Check sheet for the modelled part. Datum: model origin and axes. Units: mm. A direction names the side the tool comes from. Round coordinates to 2 decimals unless told otherwise and drop trailing zeros. Order: outer loops, then holes, each group sorted by start corner. A loop starts at its lowest first (then second) coordinate and runs counter-clockwise, first axis right, second up. Notation, with made-up numbers: (76.5, 6.5) -> (114.5, 6.5) arc R21 cw to (114.5, 14.5) -> close; hole circle Ø4 at (56.25, -19). An arc over 180 degrees is marked (long way). Answer in a Markdown table with one row per item.
```python
from build123d import *

# Parameters (mm, degrees)
F0_W         = 31
F0_H         = 21
F1_DEPTH     = 28
F2_W         = 21
F2_H         = 42
F3_DEPTH     = 50.8
F4_DEPTH     = 25.4
F6_DEPTH     = 25.4
F7_DEPTH     = 25.4
F8_DEPTH     = 2
F9_W         = 10.5
F9_H         = 2
F10_DEPTH    = 10.5
F11_DEPTH    = 10.5
F12_W        = 18.7637824565
F12_H        = 49.8975180089
F13_DEPTH    = 25.4
F14_DEPTH    = 25.4
F15_DEPTH    = 0.25
F16_DEPTH    = 0.25
F17_DEPTH    = 1
F18_T1_DEPTH = 46.4


# Not quite as in the source:
# - a fillet or chamfer that OpenCascade refuses, or shapes differently, is made with other operations: its cross-section is extruded or revolved along the edge and cut away or added


with BuildPart() as f1:
    # F0 (on Top) → F1 (new body)
    with BuildSketch(Plane.XY):
        Rectangle(F0_W, F0_H)
    extrude(amount=F1_DEPTH)

    # F2 (on Front) → F3 (cut)
    with BuildSketch(Plane.XZ):
        Rectangle(F2_W, F2_H)
    extrude(amount=-F3_DEPTH, mode=Mode.SUBTRACT)

    # F2 (on Front) → F4 (cut)
    with BuildSketch(Plane.XZ):
        Rectangle(F2_W, F2_H)
    extrude(amount=F4_DEPTH, mode=Mode.SUBTRACT)

    # F5 (on Right) → F6 (cut)
    with BuildSketch(Plane.YZ):
        with BuildLine():
            Line((0, 24.5501343161), (2.5, 24.5501343161))
            ThreePointArc((2.5, 24.5501343161), (0, 27.0501343161), (-2.5, 24.5501343161))
            Line((-2.5, 24.5501343161), (0, 24.5501343161))
        make_face()
        with BuildLine():
            Line((2.5, -28.5555105656), (2.5, 24.5501343161))
            ThreePointArc((2.5, 24.5501343161), (1.767766953, 22.7823673631), (0, 22.0501343161))
            Line((0, 22.0501343161), (0, -28.5555105656))
            Line((0, -28.5555105656), (2.5, -28.5555105656))
        make_face()
        with BuildLine():
            ThreePointArc((0, 22.0501343161), (1.767766953, 22.7823673631), (2.5, 24.5501343161))
            Line((2.5, 24.5501343161), (0, 24.5501343161))
            Line((0, 24.5501343161), (0, 22.0501343161))
        make_face()
        with BuildLine():
            Line((0, 24.5501343161), (-2.5, 24.5501343161))
            ThreePointArc((-2.5, 24.5501343161), (-1.767766953, 22.7823673631), (0, 22.0501343161))
            Line((0, 22.0501343161), (0, 24.5501343161))
        make_face()
        with BuildLine():
            ThreePointArc((0, 22.0501343161), (-1.767766953, 22.7823673631), (-2.5, 24.5501343161))
            Line((-2.5, 24.5501343161), (-2.5, -33.7370373309))
            Line((-2.5, -33.7370373309), (0, -33.7370373309))
            Line((0, -33.7370373309), (0, -28.5555105656))
            Line((0, -28.5555105656), (0, 22.0501343161))
        make_face()
    extrude(amount=-F6_DEPTH, mode=Mode.SUBTRACT)

    # F5 (on Right) → F7 (cut)
    with BuildSketch(Plane.YZ):
        with BuildLine():
            Line((0, 24.5501343161), (2.5, 24.5501343161))
            ThreePointArc((2.5, 24.5501343161), (0, 27.0501343161), (-2.5, 24.5501343161))
            Line((-2.5, 24.5501343161), (0, 24.5501343161))
        make_face()
        with BuildLine():
            Line((2.5, -28.5555105656), (2.5, 24.5501343161))
            ThreePointArc((2.5, 24.5501343161), (1.767766953, 22.7823673631), (0, 22.0501343161))
            Line((0, 22.0501343161), (0, -28.5555105656))
            Line((0, -28.5555105656), (2.5, -28.5555105656))
        make_face()
        with BuildLine():
            ThreePointArc((0, 22.0501343161), (1.767766953, 22.7823673631), (2.5, 24.5501343161))
            Line((2.5, 24.5501343161), (0, 24.5501343161))
            Line((0, 24.5501343161), (0, 22.0501343161))
        make_face()
        with BuildLine():
            Line((0, 24.5501343161), (-2.5, 24.5501343161))
            ThreePointArc((-2.5, 24.5501343161), (-1.767766953, 22.7823673631), (0, 22.0501343161))
            Line((0, 22.0501343161), (0, 24.5501343161))
        make_face()
        with BuildLine():
            ThreePointArc((0, 22.0501343161), (-1.767766953, 22.7823673631), (-2.5, 24.5501343161))
            Line((-2.5, 24.5501343161), (-2.5, -33.7370373309))
            Line((-2.5, -33.7370373309), (0, -33.7370373309))
            Line((0, -33.7370373309), (0, -28.5555105656))
            Line((0, -28.5555105656), (0, 22.0501343161))
        make_face()
    extrude(amount=F7_DEPTH, mode=Mode.SUBTRACT)

    # F8 (add): faces of the model
    f8_faces = [f1.faces().sort_by_distance(p)[0] for p in [
        (13, 6.5, 0),
        (13, -6.5, 0),
        (-13, -6.5, 0),
        (-13, 6.5, 0),
    ]]
    extrude(f8_faces, amount=F8_DEPTH)

    # F9 (on Right) → F10 (join)
    with BuildSketch(Plane.YZ):
        with Locations((-5.25, -1)):
            Rectangle(F9_W, F9_H)
        with Locations((5.25, -1)):
            Rectangle(F9_W, F9_H)
    extrude(amount=F10_DEPTH)

    # F11 (add): a face of the model
    f11_faces = [f1.faces().sort_by_distance(p)[0] for p in [
        (0, 0, -1),
    ]]
    extrude(f11_faces, amount=F11_DEPTH)

    # F12 (on Top) → F13 (cut)
    with BuildSketch(Plane.XY):
        Rectangle(F12_W, F12_H)
    extrude(amount=-F13_DEPTH, mode=Mode.SUBTRACT)

    # F14 (cut): a face of the model
    f14_faces = [f1.faces().sort_by_distance(p)[0] for p in [
        (10.5, 0, -1),
    ]]
    extrude(f14_faces, amount=-F14_DEPTH, mode=Mode.SUBTRACT)

    # F15 (add): faces of the model
    f15_faces = [f1.faces().sort_by_distance(p)[0] for p in [
        (9.3818912283, 6.5, -1),
        (9.3818912283, -6.5, -1),
    ]]
    extrude(f15_faces, amount=F15_DEPTH)

    # F16 (add): faces of the model
    f16_faces = [f1.faces().sort_by_distance(p)[0] for p in [
        (-9.3818912283, 6.5, -1),
        (-9.3818912283, -6.5, -1),
    ]]
    extrude(f16_faces, amount=F16_DEPTH)

    # F17 (add): a face of the model
    f17_faces = [f1.faces().sort_by_distance(p)[0] for p in [
        (0, 0, 28),
    ]]
    extrude(f17_faces, amount=F17_DEPTH)

    # F18: fillet of radius 5.08 on 2 edges, made by hand

    # F18_s2 → F18_t1 (cut)
    with BuildSketch(Plane.XZ.offset(-23.2)):
        with BuildLine():
            ThreePointArc((-15.5, 23.92), (-14.0121024484, 27.5121024484), (-10.42, 29))
            Line((-10.42, 29), (-15.5, 29))
            Line((-15.5, 29), (-15.5, 23.92))
        make_face()
        with BuildLine():
            ThreePointArc((15.5, 23.92), (14.0121024484, 27.5121024484), (10.42, 29))
            Line((10.42, 29), (15.5, 29))
            Line((15.5, 29), (15.5, 23.92))
        make_face()
    extrude(amount=F18_T1_DEPTH, mode=Mode.SUBTRACT)


solid = f1.part
```
(1) Section check D-D on x = -2. Record the boundary of the cut face in (y, z), plus the area to 3 significant figures.
Solutions:
| item | result |
|---|---|
| outline | (-10.5, 21) -> (-2.5, 21) -> (-2.5, 24.55) arc R2.5 cw to (2.5, 24.55) -> (2.5, 21) -> (10.5, 21) -> (10.5, 29) -> (-10.5, 29) -> close |
| area | 140 mm^2 |
(2) Tool access check on faces 5 (the flat face through (10, 6, 0)), 6 (the flat face through (0, 0, 29)), 7 (the flat face through (9.132, -7, -1)). Record the directions out of +Z, -Z, +X, -X, +Y, -Y that give a thin tool (end or side, any length) a straight path to the whole face; none if there is none.
Solutions:
| item | result |
|---|---|
| face 5 | +Y, -Y |
| face 6 | +Z, +X, -X, +Y, -Y |
| face 7 | -Z, +Y, -Y |
(3) Scan lines: probe 1 along Y at (x, z) = (12, 3); probe 2 along Z at (x, y) = (-10, 5.5); probe 3 along X at (y, z) = (-7.75, -1). Record each from-to range of solid material in increasing order. Write a range as from..to.
Solutions:
| item | result |
|---|---|
| probe 1 | -10.5..-2.5, 2.5..10.5 |
| probe 2 | -2..0, 21..29 |
| probe 3 | -15.5..-9.13, 9.13..15.5 |
(4) Draft check along Z on faces 1 (the flat face through (10.5, -6, 10)), 2 (the flat face through (-10, -6, 0)), 3 (the flat face through (9.132, 6, -1)), 4 (the flat face through (-12, -7, -2)). Enter one of: pulls with the +Z half, pulls with the -Z half, needs draft (parallel to the pull), parting line crosses it, or undercut.
Solutions:
| item | result |
|---|---|
| face 1 | undercut |
| face 2 | undercut |
| face 3 | needs draft |
| face 4 | pulls with the -Z half |
(5) Section check C-C on y = -8. Record the boundary of the cut face in (x, z), plus the area to 3 significant figures.
Solutions:
| item | result |
|---|---|
| outline | (-15.5, -2) -> (-9.13, -2) -> (-9.13, 0) -> (-10.5, 0) -> (-10.5, 21) -> (10.5, 21) -> (10.5, 0) -> (9.13, 0) -> (9.13, -2) -> (15.5, -2) -> (15.5, 23.92) arc R5.08 ccw to (10.42, 29) -> (-10.42, 29) arc R5.08 ccw to (-15.5, 23.92) -> close |
| area | 472 mm^2 |
(6) Depth check by flat-ended pin: pin 1 Ø4 at (x, y) = (-1, -6.5) entering from -Z; pin 2 Ø13.5 at (x, z) = (5.5, 17) entering from -Y. Enter the tip coordinate at first touch or a pass-through.
Solutions:
| item | result |
|---|---|
| pin 1 | z = 21 |
| pin 2 | y = -10.5 |
(7) Section check A-A on z = 17. Record the boundary of the cut face in (x, y), plus the area to 3 significant figures.
Solutions:
| item | result |
|---|---|
| outline | (-15.5, -10.5) -> (-10.5, -10.5) -> (-10.5, -2.5) -> (-15.5, -2.5) -> close; (-15.5, 2.5) -> (-10.5, 2.5) -> (-10.5, 10.5) -> (-15.5, 10.5) -> close; (10.5, -10.5) -> (15.5, -10.5) -> (15.5, -2.5) -> (10.5, -2.5) -> close; (10.5, 2.5) -> (15.5, 2.5) -> (15.5, 10.5) -> (10.5, 10.5) -> close |
| area | 160 mm^2 |
(8) Section check B-B on z = 22.5. Record the boundary of the cut face in (x, y), plus the area to 3 significant figures.
Solutions:
| item | result |
|---|---|
| outline | (-15.5, -10.5) -> (15.5, -10.5) -> (15.5, -2.5) -> (-15.5, -2.5) -> close; (-15.5, 2.5) -> (15.5, 2.5) -> (15.5, 10.5) -> (-15.5, 10.5) -> close |
| area | 496 mm^2 |
